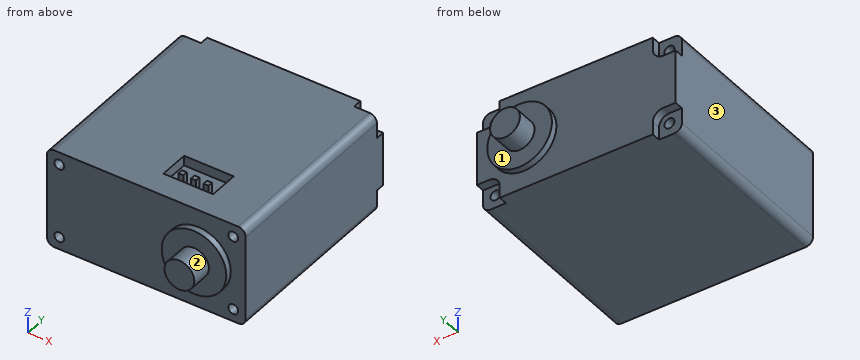
from build123d import *

# Parameters (mm, degrees)
SKETCH_1_W          = 40
SKETCH_1_H          = 20
EXTRUDE_1_DEPTH     = 20
FILLET_1_R          = 1.5
SKETCH_2_R          = 1
CUT_EXTRUDE_1_DEPTH = 41
SKETCH_3_R          = 2.1
SKETCH_3_R_2        = 1
CUT_EXTRUDE_2_DEPTH = 1.8
SKETCH_4_R          = 6.5
EXTRUDE_2_DEPTH     = 1.3
SKETCH_5_R          = 3
EXTRUDE_3_DEPTH     = 4.25
SKETCH_6_W          = 10
SKETCH_6_H          = 6
CUT_EXTRUDE_3_DEPTH = 2
SKETCH_7_W          = 1
SKETCH_7_H          = 1
EXTRUDE_4_DEPTH     = 2


with BuildPart() as part:
    # Эскиз1 → Бобышка-Вытянуть1 (new body, symmetric)
    with BuildSketch(Plane(origin=(0, 0, 0), x_dir=(1, 0, 0), z_dir=(0, 1, 0))):
        Rectangle(SKETCH_1_W, SKETCH_1_H)
    extrude(amount=EXTRUDE_1_DEPTH, both=True)

    # Скругление1
    fillet_1_edges = [part.edges().sort_by_distance(p)[0] for p in [
        (20, 0, 10),
        (-20, 0, 10),
        (-20, 0, -10),
        (20, 0, -10),
    ]]
    fillet(fillet_1_edges, radius=FILLET_1_R)

    # Эскиз2 → Вырез-Вытянуть1 (cut, through all)
    with BuildSketch(Plane(origin=(0, 20, 0), x_dir=(1, 0, 0), z_dir=(0, 1, 0))):
        with Locations((17.5, 7.5)):
            Circle(SKETCH_2_R)
        with Locations((17.5, -7.5)):
            Circle(SKETCH_2_R)
        with Locations((-17.5, -7.5)):
            Circle(SKETCH_2_R)
        with Locations((-17.5, 7.5)):
            Circle(SKETCH_2_R)
    extrude(amount=-CUT_EXTRUDE_1_DEPTH, mode=Mode.SUBTRACT)

    # Эскиз3 → Вырез-Вытянуть2 (cut)
    with BuildSketch(Plane(origin=(0, 20, 0), x_dir=(1, 0, 0), z_dir=(0, 1, 0))):
        with Locations((-17.5, 7.5)):
            Circle(SKETCH_3_R)
        with Locations((-17.5, 7.5)):
            Circle(SKETCH_3_R_2, mode=Mode.SUBTRACT)
        with BuildLine():
            Line((-20, 8.5), (-20, 5.4))
            Line((-20, 5.4), (-17.5, 5.4))
            ThreePointArc((-17.5, 5.4), (-18.98492424, 8.98492424), (-15.4, 7.5))
            Line((-15.4, 7.5), (-15.4, 10))
            Line((-15.4, 10), (-18.5, 10))
            ThreePointArc((-18.5, 10), (-19.560660172, 9.560660172), (-20, 8.5))
        make_face()
        with Locations((-17.5, -7.5)):
            Circle(SKETCH_3_R)
        with Locations((-17.5, -7.5)):
            Circle(SKETCH_3_R_2, mode=Mode.SUBTRACT)
        with BuildLine():
            Line((-17.5, -5.4), (-20, -5.4))
            Line((-20, -5.4), (-20, -8.5))
            ThreePointArc((-20, -8.5), (-19.560660172, -9.560660172), (-18.5, -10))
            Line((-18.5, -10), (-15.4, -10))
            Line((-15.4, -10), (-15.4, -7.5))
            ThreePointArc((-15.4, -7.5), (-18.98492424, -8.98492424), (-17.5, -5.4))
        make_face()
        with BuildLine():
            Line((15.4, -7.499999992), (15.4, -10))
            Line((15.4, -10), (18.5, -10))
            ThreePointArc((18.5, -10), (19.560660172, -9.560660172), (20, -8.5))
            Line((20, -8.5), (20, -5.4))
            Line((20, -5.4), (17.5, -5.4))
            ThreePointArc((17.5, -5.4), (18.98492424, -6.01507576), (19.6, -7.5))
            ThreePointArc((19.6, -7.5), (17.499999996, -9.6), (15.4, -7.499999992))
        make_face()
        with Locations((17.5, -7.5)):
            Circle(SKETCH_3_R)
        with Locations((17.5, -7.5)):
            Circle(SKETCH_3_R_2, mode=Mode.SUBTRACT)
        with BuildLine():
            Line((18.5, 10), (15.4, 10))
            Line((15.4, 10), (15.4, 7.500000012))
            ThreePointArc((15.4, 7.500000012), (17.500000006, 9.6), (19.6, 7.5))
            ThreePointArc((19.6, 7.5), (18.98492424, 6.01507576), (17.5, 5.4))
            Line((17.5, 5.4), (20, 5.4))
            Line((20, 5.4), (20, 8.5))
            ThreePointArc((20, 8.5), (19.560660172, 9.560660172), (18.5, 10))
        make_face()
        with Locations((17.5, 7.5)):
            Circle(SKETCH_3_R)
        with Locations((17.5, 7.5)):
            Circle(SKETCH_3_R_2, mode=Mode.SUBTRACT)
    extrude(amount=-CUT_EXTRUDE_2_DEPTH, mode=Mode.SUBTRACT)

    # Эскиз4 → Бобышка-Вытянуть2 (add)
    with BuildSketch(Plane(origin=(0, 20, 0), x_dir=(1, 0, 0), z_dir=(0, 1, 0))):
        with Locations((10.5, 0)):
            Circle(SKETCH_4_R)
    extrude_2 = extrude(amount=EXTRUDE_2_DEPTH)

    # Эскиз5 → Бобышка-Вытянуть3 (add)
    with BuildSketch(Plane(origin=(0, 21.3, 0), x_dir=(1, 0, 0), z_dir=(0, 1, 0))):
        with Locations((10.5, 0)):
            Circle(SKETCH_5_R)
    extrude_3 = extrude(amount=EXTRUDE_3_DEPTH)

    # Зеркальное отражение1: Бобышка-Вытянуть2, Бобышка-Вытянуть3 across plane
    add(extrude_2.mirror(Plane.ZX))
    add(extrude_3.mirror(Plane.ZX))

    # Эскиз6 → Вырез-Вытянуть3 (cut)
    with BuildSketch(Plane.XY.offset(10)):
        with Locations((5, -12)):
            Rectangle(SKETCH_6_W, SKETCH_6_H)
    extrude(amount=-CUT_EXTRUDE_3_DEPTH, mode=Mode.SUBTRACT)

    # Эскиз7 → Бобышка-Вытянуть4 (add)
    with BuildSketch(Plane.XY.offset(8)):
        with Locations((2.46, -13)):
            Rectangle(SKETCH_7_W, SKETCH_7_H)
        with Locations((5, -13)):
            Rectangle(SKETCH_7_W, SKETCH_7_H)
        with Locations((7.54, -13)):
            Rectangle(SKETCH_7_W, SKETCH_7_H)
    extrude(amount=EXTRUDE_4_DEPTH)


solid = part.part
Source: CAD feature listing. Evaluate the final solid. Frame: model axes, mm. Face numbers are marked on the shaded views. A direction names the side the tool comes from. Round coordinates to 2 decimals unless told otherwise and drop trailing zeros. Loops run counter-clockwise (first coordinate to the right, second up) from the corner with the lowest first, then second, coordinate; pieces in that order, holes last. Notation, with made-up numbers: M 4.25,-35 L 62.25,-35 A14 ccw 62.25,-11 Z; hole C 44.25,-20 d5. An arc over 180 degrees is marked long. Return JSON: item names as keys, results as strings. Group by question number.
1. Section query B-B on z = 0. Output: boundary loops of the cut face in (x, y), and give its area (3 significant figures).
2. Section query A-A on y = -3. Output: boundary loops of the cut face in (x, z).
3. Reachability of the marked faces 1, 2 and 3 from +Z, -Z, +X, -X, +Y, -Y: full face, straight path, thin tool, end or side. Return the list, or none.
4. Section query C-C on y = 22.5. Output: boundary loops of the cut face in (x, z), and give its area (3 significant figures).
5. Pin query (flat end, axial travel): pin 1 (0.5 mm diameter, centred on y = -13, z = 9.5, fed in from -X); pin 2 (3 mm diameter, centred on x = -17.5, z = 7.5, fed in from -Y); pin 3 (0.5 mm diameter, centred on y = -13, z = 9, fed in from +X). Return the tip coordinate at first contact, or that it passes through.
6. Material intervals for line 1 along Z through (x, y) = (-17.5, -0.5); line 2 along X through (y, z) = (-10, -7.5); line 3 along Y through (x, z) = (6.5, 0.25), sorted ascending. Write a range as from..to.
Checks:
{
 "1": {"outline": "M -20,-20 L 4,-20 L 4,-21.3 L 7.5,-21.3 L 7.5,-25.55 L 13.5,-25.55 L 13.5,-21.3 L 17,-21.3 L 17,-20 L 20,-20 L 20,20 L 17,20 L 17,21.3 L 13.5,21.3 L 13.5,25.55 L 7.5,25.55 L 7.5,21.3 L 4,21.3 L 4,20 L -20,20 Z", "area": "1,680 mm²"},
 "2": {"outline": "M -20,-8.5 A1.5 ccw -18.5,-10 L 18.5,-10 A1.5 ccw 20,-8.5 L 20,8.5 A1.5 ccw 18.5,10 L -18.5,10 A1.5 ccw -20,8.5 Z; hole C -17.5,-7.5 d2; hole C -17.5,7.5 d2; hole C 17.5,-7.5 d2; hole C 17.5,7.5 d2"},
 "3": {"face 1": "+Y", "face 2": "-Y", "face 3": "+Z, -Z, -X, +Y, -Y"},
 "4": {"outline": "C 10.5,0 d6", "area": "28.3 mm²"},
 "5": {"pin 1": "stops at x = -19.8", "pin 2": "stops at y = -20", "pin 3": "stops at x = 19.98"},
 "6": {"line 1": "z = -10..-8.5, -6.5..6.5, 8.5..10", "line 2": "x = -20..-18.5, -16.5..16.5, 18.5..20", "line 3": "y = -21.3..21.3"}
}
